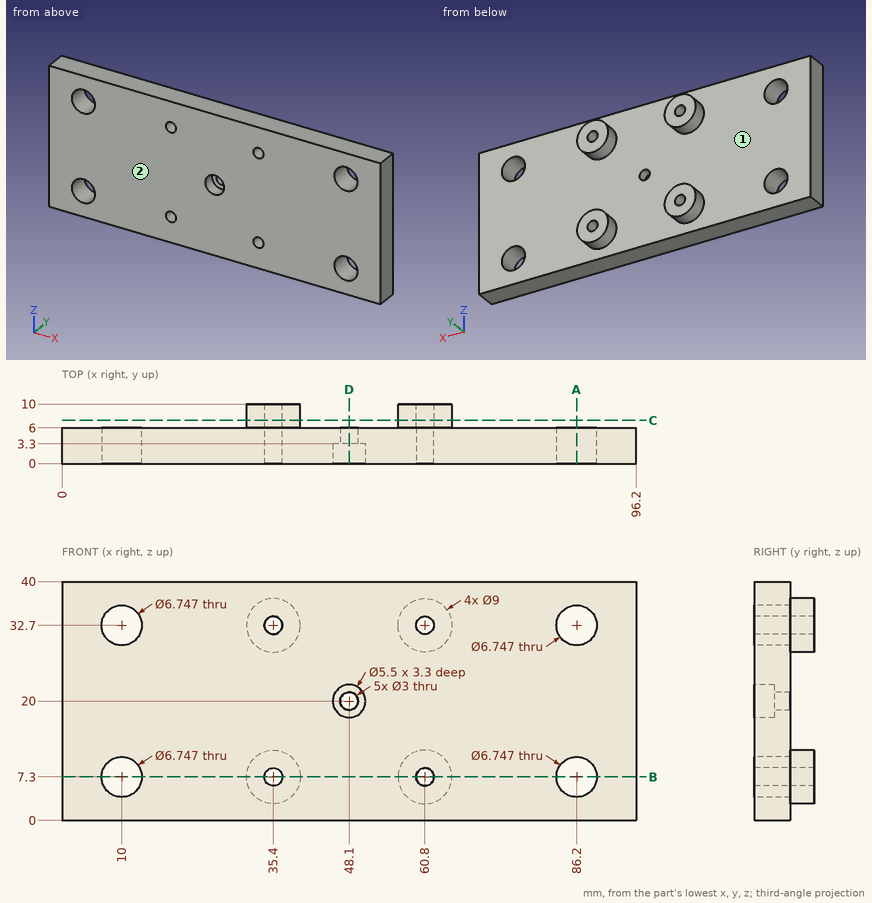
Design review of the part shown in the three views and the two pictorial views. Dimensions are in mm from the part's minimum x, y and z. A direction names the side the tool comes from. Give positions to 0.01 mm unless a question says otherwise; leave off trailing zeros. Loops run counter-clockwise (first coordinate to the right, second up) from the corner with the lowest first, then second, coordinate; pieces in that order, holes last. Notation, with made-up numbers: (27, 83.5) - (51, 83.5) arc R31 cw to (51, 116.5) - close; hole circle Ø7 at (30.5, -27). An arc over 180 degrees is marked (long way). Use CSV: the item, a comma, the result in double quotes. Start each with the question number.
1. Wall thickness on L1, parallel to Z at x = 35.4, y = 3; L2, parallel to Z at x = 86.2, y = 4.65; L3, parallel to X at y = 4.25, z = 7.5: over which ranges is each line inside the solid? List them lowest first.
2. Add section C-C (y = 7.25). State the section outline as (x, z) points.
3. Insertion check: P1, Ø8, axis at x = 86.2, z = 32.7, coming from the -Y side; P2, Ø2.5, axis at x = 60.8, z = 7.3, coming from the -Y side; P3, Ø3, axis at y = 8.5, z = 7, coming from the +X side; P4, Ø3.5, axis at x = 48.1, z = 20, coming from the -Y side. Each pin has a flat end and moves straight along its axis. Give the tip position at first contact, or say it passes through.
4. Add section D-D (x = 48.1). State the section outline as (y, z) points, plus the area to 3 significant figures.
5. Machinability: for the marked faces 1 and 2, which of the approach directions +Z, -Z, +X, -X, +Y, -Y give a long, thin tool a straight path to every point of the face, cutting with its end or side? Answer none if there is none.
6. Add section A-A (x = 86.2). State the section outline as (y, z) points, plus the area to 3 significant figures.
7. Add section B-B (z = 7.3). State the section outline as (x, y) points.
Results found:
1,L1,"z = 0 to 5.8, 8.8 to 31.2, 34.2 to 40"
1,L2,"z = 0 to 3.93, 10.67 to 29.33, 36.07 to 40"
1,L3,"x = 0 to 6.63, 13.37 to 33.91, 36.89 to 59.31, 62.29 to 82.83, 89.57 to 96.2"
2,outline,"circle Ø9 at (35.4, 7.3); circle Ø9 at (35.4, 32.7); circle Ø9 at (60.8, 7.3); circle Ø9 at (60.8, 32.7); hole circle Ø3 at (35.4, 7.3); hole circle Ø3 at (35.4, 32.7); hole circle Ø3 at (60.8, 7.3); hole circle Ø3 at (60.8, 32.7)"
3,P1,"stops at y = 0"
3,P2,"passes through"
3,P3,"stops at x = 65.3"
3,P4,"stops at y = 3.3"
4,outline,"(0, 0) - (6, 0) - (6, 18.5) - (3.3, 18.5) - (3.3, 17.25) - (0, 17.25) - close; (0, 22.75) - (3.3, 22.75) - (3.3, 21.5) - (6, 21.5) - (6, 40) - (0, 40) - close"
4,area,"214 mm²"
5,face 1,"+Y"
5,face 2,"+Z, -Z, +X, -X, -Y"
6,outline,"(0, 0) - (6, 0) - (6, 3.93) - (0, 3.93) - close; (0, 10.67) - (6, 10.67) - (6, 29.33) - (0, 29.33) - close; (0, 36.07) - (6, 36.07) - (6, 40) - (0, 40) - close"
6,area,"159 mm²"
7,outline,"(0, 0) - (6.63, 0) - (6.63, 6) - (0, 6) - close; (13.37, 0) - (33.9, 0) - (33.9, 10) - (30.9, 10) - (30.9, 6) - (13.37, 6) - close; (36.9, 0) - (59.3, 0) - (59.3, 10) - (56.3, 10) - (56.3, 6) - (39.9, 6) - (39.9, 10) - (36.9, 10) - close; (62.3, 0) - (82.83, 0) - (82.83, 6) - (65.3, 6) - (65.3, 10) - (62.3, 10) - close; (89.57, 0) - (96.2, 0) - (96.2, 6) - (89.57, 6) - close"
